The model under review builds one solid part; all positions refer to its coordinate system, in mm. A direction names the side the tool comes from. Coordinates: 2 decimals unless noted, no trailing zeros. Order: outer loops, then holes, each group sorted by start corner. A loop starts at its lowest first (then second) coordinate and runs counter-clockwise, first axis right, second up. Notation, with made-up numbers: (-5, 79) -> (8, 79) arc R24 cw to (8, 101) -> close; hole circle Ø6 at (52, 83). An arc over 180 degrees is marked (long way). Put each result on its own line as item: value.
from build123d import *

# Parameters (mm, degrees)
F0_W     = 9.525
F0_H     = 28.575
F0_R     = 2.15265
F1_DEPTH = 36.195
F2_R     = 2.15265
F3_DEPTH = 9.525
F4_R     = 4.7625
F5_W     = 11.45515
F5_H     = 3.175
F6_DEPTH = 25.4
F8_DEPTH = 3.175


with BuildPart() as f1:
    # F0 (on Top) → F1 (new body)
    with BuildSketch(Plane.XY):
        with Locations((-4.7625, -14.2875)):
            Rectangle(F0_W, F0_H)
        with Locations((-4.7625, -23.8125)):
            Circle(F0_R, mode=Mode.SUBTRACT)
        with Locations((-4.7625, -4.7625)):
            Circle(F0_R, mode=Mode.SUBTRACT)
    extrude(amount=F1_DEPTH)

    # F2 (on face) → F3 (cut, through all)
    with BuildSketch(Plane.YZ):
        with Locations((-14.2875, 31.4325)):
            Circle(F2_R)
        with Locations((-14.2875, 4.7625)):
            Circle(F2_R)
    extrude(amount=-F3_DEPTH, mode=Mode.SUBTRACT)

    # F4
    f4_edges = [f1.edges().sort_by_distance(p)[0] for p in [
        (0, -28.575, 18.0975),
        (0, 0, 18.0975),
    ]]
    fillet(f4_edges, radius=F4_R)

    # F5 (on face) → F6 (join)
    with BuildSketch(Plane(origin=(-9.525, 0, 0), x_dir=(0, -1, 0), z_dir=(-1, 0, 0))):
        with Locations((14.2875, 25.0825)):
            Rectangle(F5_W, F5_H)
    extrude(amount=F6_DEPTH)

    # F7 (on face) → F8 (cut, through all)
    with BuildSketch(Plane.XY.offset(26.67)):
        Polygon((-12.7, -8.559925), (-34.925, -8.559925), (-34.925, -20.015075), (-12.7, -20.015075), (-17.077984, -16.377956), (-17.077984, -12.197044), align=None)
    extrude(amount=-F8_DEPTH, mode=Mode.SUBTRACT)


solid = f1.part
Item 1: For faces 5 (the flat face through (-5, -14, 0)), 6 (the flat face through (-12, -14, 26.67)), 7 (the flat face through (-11, -8.56, 25)), 8 (the flat face through (-11, -20.015, 25)), 9 (the flat face through (-7, 0, 18)), list the 3-axis set-ups (+Z, -Z, +X, -X, +Y, -Y) from which the entire face can be reached by the end or side of a thin tool; tool diameter is ignored.
Answers below:
face 5: -Z, +X, -X, +Y, -Y
face 6: +Z, -X, +Y, -Y
face 7: +Z, -Z, -X, +Y
face 8: +Z, -Z, -X, -Y
face 9: +Z, -Z, +X, -X, +Y
Item 2: For pin 1 Ø5.5 at (x, y) = (-4.76, -4.76) entering from +Z (3 decimals); pin 2 Ø12 at (y, z) = (-23.5, 25.5) entering from -X; pin 3 Ø2.5 at (x, y) = (-12.5, -14.5) entering from +Z; pin 4 Ø1 at (x, z) = (-11.5, 25) entering from -Y, all flat-tipped, find the tip position at first contact; note any pin that passes through.
Answers below:
pin 1: z = 36.195
pin 2: x = -15.73
pin 3: z = 26.67
pin 4: y = -20.02
Item 3: Consider section C-C on y = -22.5. Write out the cut boundary in (x, z) (3 decimals).
Answers below:
outline: (-9.525, 0) -> (-6.469, 0) -> (-6.469, 36.195) -> (-9.525, 36.195) -> close; (-3.056, 0) -> (0, 0) -> (0, 36.195) -> (-3.056, 36.195) -> close
Item 4: Consider section A-A on z = 32. Write out the cut boundary in (x, y) (1 decimal).
Answers below:
outline: (-9.5, -28.6) -> (-4.8, -28.6) arc R4.8 ccw to (0, -23.8) -> (0, -16.4) -> (-9.5, -16.4) -> close; (-9.5, -12.2) -> (0, -12.2) -> (0, -4.8) arc R4.8 ccw to (-4.8, 0) -> (-9.5, 0) -> close; hole circle Ø4.3 at (-4.8, -23.8); hole circle Ø4.3 at (-4.8, -4.8)
Item 5: Mouldability with a two-part tool opening along X and no side actions: class faces 1 (the flat face through (-12, -14, 23.495)), 2 (the flat face through (0, -14, 18)), 3 (the cylindrical face through (-5.043, -21.678, 17.844)), 4 (the cylindrical face through (-5.229, -6.864, 17.844)) as +X half, -X half, draft (parallel to the pull), parting line (faces both ways), or undercut.
Answers below:
face 1: draft
face 2: +X half
face 3: undercut
face 4: undercut
Item 6: For line 1 (Y direction, x = -3.25, z = 10); line 2 (Y direction, x = -4.5, z = 27); line 3 (Z direction, x = -2.5, y = -15.5) (3 decimals), list the stretches that pass through material, from the lowest coordinate up. Write a range as from..to.
Answers below:
line 1: -28.33..-25.34, -22.28..-6.29, -3.23..-0.25
line 2: -28.57..-25.95, -21.68..-6.9, -2.63..-0.01
line 3: 0..2.984, 6.541..29.654, 33.211..36.195
Item 7: Consider section B-B on x = -6. Write out the cut boundary in (y, z) (1 decimal).
Answers below:
outline: (-28.6, 0) -> (-25.6, 0) -> (-25.6, 36.2) -> (-28.6, 36.2) -> close; (-22.1, 0) -> (-6.5, 0) -> (-6.5, 36.2) -> (-22.1, 36.2) -> close; (-3, 0) -> (0, 0) -> (0, 36.2) -> (-3, 36.2) -> close; hole circle Ø4.3 at (-14.3, 4.8); hole circle Ø4.3 at (-14.3, 31.4)
Item 8: Consider section D-D on z = 13. Write out the cut boundary in (x, y) (1 decimal), and give its area (3 significant figures).
Answers below:
outline: (-9.5, -28.6) -> (-4.8, -28.6) arc R4.8 ccw to (0, -23.8) -> (0, -4.8) arc R4.8 ccw to (-4.8, 0) -> (-9.5, 0) -> close; hole circle Ø4.3 at (-4.8, -23.8); hole circle Ø4.3 at (-4.8, -4.8)
area: 233 mm^2
